Study the drawing (mm; zero at the part's minimum x, y, z) and answer. Coordinates: 2 decimals unless noted, no trailing zeros. Write each loop counter-clockwise with the first axis right and the second up, starting at its lowest first coordinate (ties: lowest second). Pieces come first, ordered by that corner, then holes. Notation, with made-up numbers: (1.5, 47.5) - (60.5, 47.5) arc R33 cw to (60.5, 82.5) - close; hole circle Ø6 at (88, 28). An arc over 180 degrees is marked (long way). One line per item, written item: value.
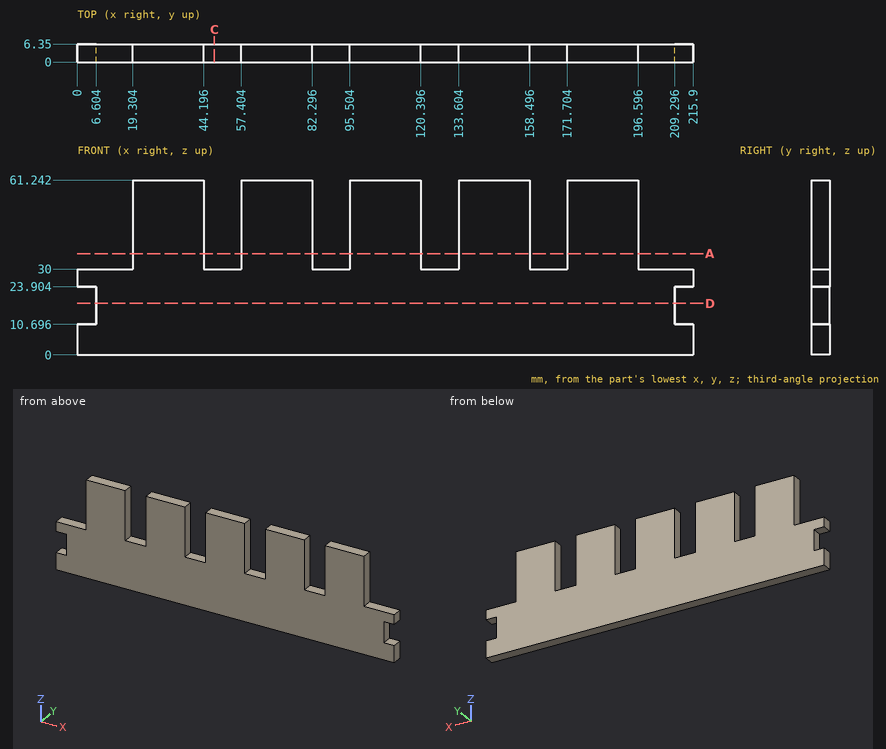
Item 1: Section A-A, the plane z = 35.5 is taken. Determine the outline of the cut face in (x, y), then the cut area to 3 significant figures.
Evaluation:
outline: (19.3, 0) - (44.2, 0) - (44.2, 6.35) - (19.3, 6.35) - close; (57.4, 0) - (82.3, 0) - (82.3, 6.35) - (57.4, 6.35) - close; (95.5, 0) - (120.4, 0) - (120.4, 6.35) - (95.5, 6.35) - close; (133.6, 0) - (158.5, 0) - (158.5, 6.35) - (133.6, 6.35) - close; (171.7, 0) - (196.6, 0) - (196.6, 6.35) - (171.7, 6.35) - close
area: 790 mm2
Item 2: Consider probe 1 along X at (y, z) = (3, 47); probe 2 along Z at (x, y) = (94.5, 2). Determine where each line is inside the solid, lowest interval first.
Evaluation:
probe 1: x = 19.3 to 44.2, 57.4 to 82.3, 95.5 to 120.4, 133.6 to 158.5, 171.7 to 196.6
probe 2: z = 0 to 30
Item 3: Section D-D, the plane z = 18 is taken. Determine the outline of the cut face in (x, y).
Evaluation:
outline: (6.6, 0) - (209.3, 0) - (209.3, 6.35) - (6.6, 6.35) - close
Item 4: Given pin 1 (1.9 mm diameter, centred on y = 3.5, z = 44.5, fed in from -X); pin 2 (3 mm diameter, centred on y = 2.5, z = 43.5, fed in from +X); pin 3 (1.9 mm diameter, centred on x = 51.5, y = 2, fed in from +Z), each flat-ended and moving along its own axis, determine where each tip first touches the part or whether it passes through.
Evaluation:
pin 1: stops at x = 19.3
pin 2: stops at x = 196.6
pin 3: stops at z = 30
Item 5: Section C-C, the plane x = 48 is taken. Determine the outline of the cut face in (y, z), then the cut area to 4 significant figures.
Evaluation:
outline: (0, 0) - (6.35, 0) - (6.35, 30) - (0, 30) - close
area: 190.5 mm2
